Can you work these out from the model? Positions are in its coordinate system, mm. Coordinates: 2 decimals unless noted, no trailing zeros. Loops run counter-clockwise (first coordinate to the right, second up) from the corner with the lowest first, then second, coordinate; pieces in that order, holes last.
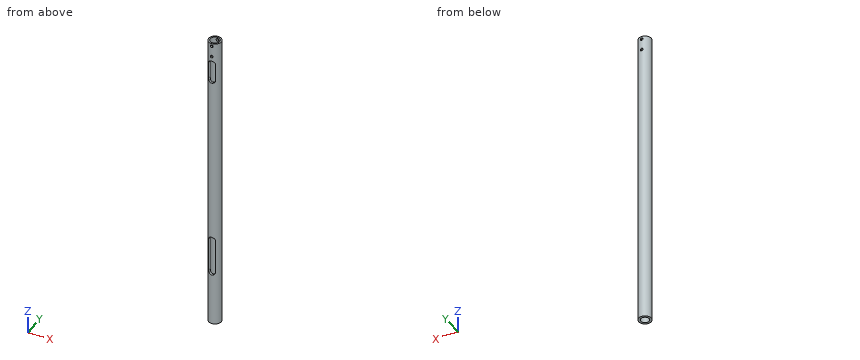
```python
from build123d import *

# Parameters (mm, degrees)
SKETCH1_R                            = 14.2875
SKETCH1_R_2                          = 9.525
BOSS_EXTRUDE1_DEPTH                  = 685.8
CUT_EXTRUDE1_DEPTH                   = 687.097591682
CUT_EXTRUDE2_START                   = -38.1
SKETCH3_R                            = 10.795
SKETCH3_R_2                          = 9.525
CUT_EXTRUDE2_DEPTH                   = 38.1
CUT_EXTRUDE3_DEPTH                   = 687.097591787
SKETCH7_W                            = 3.175
SKETCH7_H                            = 14.2875
F_1_4_0_25_DIAMETER_HOLE1_AT_2_COUNT = 2
F_1_4_0_25_DIAMETER_HOLE1_AT_2_PITCH = 25.4
CIRPATTERN1_COUNT                    = 2
CIRPATTERN1_COPY_1_SKETCH_W          = 3.175
CIRPATTERN1_COPY_1_SKETCH_H          = 14.2875


with BuildPart() as part:
    # Sketch1 → Boss-Extrude1 (new body)
    with BuildSketch(Plane.XY):
        Circle(SKETCH1_R)
        Circle(SKETCH1_R_2, mode=Mode.SUBTRACT)
    extrude(amount=BOSS_EXTRUDE1_DEPTH)

    # Sketch2 → Cut-Extrude1 (cut, through all)
    with BuildSketch(Plane(origin=(0, 0, 0), x_dir=(1, 0, 0), z_dir=(0, 1, 0))):
        with BuildLine():
            Line((7.9375, -127), (7.9375, -203.2))
            ThreePointArc((7.9375, -203.2), (0, -211.1375), (-7.9375, -203.2))
            Line((-7.9375, -203.2), (-7.9375, -127))
            ThreePointArc((-7.9375, -127), (0, -119.0625), (7.9375, -127))
        make_face()
    extrude(amount=-CUT_EXTRUDE1_DEPTH, mode=Mode.SUBTRACT)

    # Sketch3 → Cut-Extrude2 (cut)
    with BuildSketch(Plane.XY.offset(685.8).offset(CUT_EXTRUDE2_START)):
        Circle(SKETCH3_R)
        Circle(SKETCH3_R_2, mode=Mode.SUBTRACT)
    extrude(amount=CUT_EXTRUDE2_DEPTH, mode=Mode.SUBTRACT)

    # Sketch4 → Cut-Extrude3 (cut, through all)
    with BuildSketch(Plane(origin=(0, 0, 0), x_dir=(1, 0, 0), z_dir=(0, 1, 0))):
        with BuildLine():
            Line((-8.001, -635), (-8.001, -596.9))
            ThreePointArc((-8.001, -596.9), (0, -588.899), (8.001, -596.9))
            Line((8.001, -596.9), (8.001, -635))
            ThreePointArc((8.001, -635), (0, -643.001), (-8.001, -635))
        make_face()
    extrude(amount=-CUT_EXTRUDE3_DEPTH, mode=Mode.SUBTRACT)

    # Sketch7 → 1/4 (0.25) Diameter Hole1 (revolve, cut)
    with BuildSketch(Plane(origin=(0, 0, 654.05), x_dir=(0, 0, -1), z_dir=(1, 0, 0))):
        with Locations((1.5875, 7.14375)):
            Rectangle(SKETCH7_W, SKETCH7_H)
    f_1_4_0_25_diameter_hole1 = revolve(axis=Axis((0, -6.35, 654.05), (0, 1, 0)), mode=Mode.SUBTRACT)

    # 1/4 (0.25) Diameter Hole1 at 2: 1/4 (0.25) Diameter Hole1 ×2
    with Locations(*[(0, 0, i * F_1_4_0_25_DIAMETER_HOLE1_AT_2_PITCH) for i in range(1, F_1_4_0_25_DIAMETER_HOLE1_AT_2_COUNT)]):
        add(f_1_4_0_25_diameter_hole1, mode=Mode.SUBTRACT)

    # CirPattern1: 1/4 (0.25) Diameter Hole1 ×2 about axis
    cirpattern1_axis = Axis((0, 0, 647.7), (0, 0, 1))
    for i in range(1, CIRPATTERN1_COUNT):
        add(f_1_4_0_25_diameter_hole1.rotate(cirpattern1_axis, i * 360 / CIRPATTERN1_COUNT), mode=Mode.SUBTRACT)

    # CirPattern1 copy 1 sketch → CirPattern1 copy 1 (revolve, cut)
    with BuildSketch(Plane(origin=(0, 0, 679.45), x_dir=(0, 0, -1), z_dir=(-1, 0, 0))):
        with Locations((1.5875, 7.14375)):
            Rectangle(CIRPATTERN1_COPY_1_SKETCH_W, CIRPATTERN1_COPY_1_SKETCH_H)
    revolve(axis=Axis((0, 6.35, 679.45), (0, -1, 0)), mode=Mode.SUBTRACT)


solid = part.part
```
(1) I'm going to push flat-ended pins straight in: pin 1 (17 mm diameter, centred on x = 0, y = 0, fed in from +Z); pin 2 (1 mm diameter, centred on x = -4, z = 441.5, fed in from +Y); pin 3 (2 mm diameter, centred on y = -7, z = 164, fed in from +X); pin 4 (7.5 mm diameter, centred on y = -8, z = 617, fed in from -X). Where does each tip first touch, or does it pass through?
Check values:
pin 1: passes through
pin 2: stops at y = 13.85
pin 3: stops at x = 12.97
pin 4: stops at x = -13.64
(2) I want a section at A-A on y = 0. Write out the boundary of the cut face in (x, z) (1 decimal).
Check values:
outline: (-14.3, 0) - (-9.5, 0) - (-9.5, 647.7) - (-10.8, 647.7) - (-10.8, 685.8) - (-14.3, 685.8) - close; (9.5, 0) - (14.3, 0) - (14.3, 685.8) - (10.8, 685.8) - (10.8, 647.7) - (9.5, 647.7) - close
(3) If I drill on probe 1 along Z at (x, y) = (0, -12.8) (1 decimal); probe 2 along Z at (x, y) = (0, 11.95) (3 decimals); probe 3 along Y at (x, z) = (0, 485) (1 decimal), over which ranges is the centre line in solid material (lowest first)?
Check values:
probe 1: z = 0 to 119.1, 211.1 to 588.9, 643 to 650.9, 657.2 to 676.3, 682.6 to 685.8
probe 2: z = 0 to 650.875, 657.225 to 676.275, 682.625 to 685.8
probe 3: y = -14.3 to -9.5, 9.5 to 14.3
